from build123d import *

# Parameters (mm, degrees)
SKETCH1_W               = 10.16
SKETCH1_H               = 3.175
BOSS_EXTRUDE1_DEPTH     = 4.445
SKETCH3_OUTSIDE_W       = 14.934
SKETCH3_OUTSIDE_H       = 13.664
SKETCH3_OUTSIDE_W_2     = 10.16
SKETCH3_OUTSIDE_H_2     = 8.89
SKETCH3_OUTSIDE_W_3     = 5.08
SKETCH3_OUTSIDE_H_3     = 5.08
CUT_EXTRUDE1_DEPTH      = 1.905
CUT_EXTRUDE2_DEPTH      = 1
CUT_EXTRUDE2_DEPTH_BACK = 4.175
SKETCH6_R               = 1.5875
CUT_EXTRUDE3_DEPTH      = 0.2032


with BuildPart() as part:
    # Sketch1 → Boss-Extrude1 (new body, symmetric)
    with BuildSketch(Plane.XY):
        with Locations((0, -1.5875)):
            Rectangle(SKETCH1_W, SKETCH1_H)
    extrude(amount=BOSS_EXTRUDE1_DEPTH, both=True)

    # Sketch3 outside → Cut-Extrude1 (cut)
    with BuildSketch(Plane.XZ.offset(3.175)):
        Rectangle(SKETCH3_OUTSIDE_W, SKETCH3_OUTSIDE_H)
        Rectangle(SKETCH3_OUTSIDE_W_2, SKETCH3_OUTSIDE_H_2, mode=Mode.SUBTRACT)
        Rectangle(SKETCH3_OUTSIDE_W_3, SKETCH3_OUTSIDE_H_3)
    extrude(amount=-CUT_EXTRUDE1_DEPTH, mode=Mode.SUBTRACT)

    # Sketch5 → Cut-Extrude2 (cut, two sides)
    with BuildSketch(Plane(origin=(0, 0, 0), x_dir=(1, 0, 0), z_dir=(0, 1, 0))) as cut_extrude2_sk:
        with BuildLine():
            Line((0, 4.445), (-5.08, 4.445))
            Line((-5.08, 4.445), (-5.08, -4.445))
            Line((-5.08, -4.445), (0, -4.445))
            ThreePointArc((0, -4.445), (-4.445, 0), (0, 4.445))
        make_face()
    extrude(amount=CUT_EXTRUDE2_DEPTH, mode=Mode.SUBTRACT)
    extrude(cut_extrude2_sk.sketch, amount=-CUT_EXTRUDE2_DEPTH_BACK, mode=Mode.SUBTRACT)

    # Sketch6 → Cut-Extrude3 (cut)
    with BuildSketch(Plane.XZ.offset(1.27)):
        Circle(SKETCH6_R)
    extrude(amount=-CUT_EXTRUDE3_DEPTH, mode=Mode.SUBTRACT)


solid = part.part
Can you work these out from the model? Positions are in its coordinate system, mm. A direction names the side the tool comes from. Round coordinates to 2 decimals unless told otherwise and drop trailing zeros. Write each loop counter-clockwise with the first axis right and the second up, starting at its lowest first coordinate (ties: lowest second). Pieces come first, ordered by that corner, then holes. Notation, with made-up numbers: M 78.5,59 L 137.5,59 A21 cw 137.5,77 Z; hole C 72.25,15 d10. An arc over 180 degrees is marked long. Use a Markdown table: item, result.
Item 1: We'd pull the mould along X, two halves only. Please class faces 1 (the face through (-4.444, -1.565, 0.098)), 2 (the face through (3, -2, 4.445)), 3 (the face through (-2.54, -2, 0)): released by +X, released by -X, zero draft, split by the parting line, or undercut.
Found:
| item | result |
|---|---|
| face 1 | released by -X |
| face 2 | zero draft |
| face 3 | undercut |
Item 2: For pin 1 Ø2.5 at (x, z) = (-0.5, 0.5) entering from -Y; pin 2 Ø1.6 at (x, z) = (-0.5, 0.5) entering from -Y; pin 3 Ø0.6 at (x, y) = (-1, -2.5) entering from +Z, each with a flat end and sliding along its axis, tell me the tip position at first contact or that it passes through.
Found:
| item | result |
|---|---|
| pin 1 | stops at y = -1.27 |
| pin 2 | stops at y = -1.07 |
| pin 3 | stops at z = 4.39 |
Item 3: Which directions (+Z, -Z, +X, -X, +Y, -Y) give clear straight access to the entire face, cutting with the end or side of a thin tool? Please do faces 4 (the face through (0, -2, 2.54)), 5 (the face through (0, 0, 0)).
Found:
| item | result |
|---|---|
| face 4 | -Y |
| face 5 | +Z, -Z, +X, -X, +Y |
Item 4: If I drill on line 1 along X through (y, z) = (-2.65, -1); line 2 along X through (y, z) = (-2.8, 0.75); line 3 along Z through (x, y) = (-1.75, -2.1), over which ranges is the centre line in solid material (lowest first)? Write a range as [from, to].
Found:
| item | result |
|---|---|
| line 1 | x = [-4.33, -2.54], [2.54, 5.08] |
| line 2 | x = [-4.38, -2.54], [2.54, 5.08] |
| line 3 | z = [-4.09, -2.54], [2.54, 4.09] |
Item 5: I want a section at C-C (x = -0.5). List the corners of the cut face in (y, z) for me (3 decimals), and give its area (3 significant figures).
Found:
| item | result |
|---|---|
| outline | M -3.175,-4.417 L 0,-4.417 L 0,4.417 L -3.175,4.417 L -3.175,2.54 L -1.27,2.54 L -1.27,1.507 L -1.067,1.507 L -1.067,-1.507 L -1.27,-1.507 L -1.27,-2.54 L -3.175,-2.54 Z |
| area | 17.8 mm2 |
Item 6: I want a section at A-A (y = -1.75). List the corners of the cut face in (x, z) for me (3 decimals), and give its area (3 significant figures).
Found:
| item | result |
|---|---|
| outline | M 0,-4.445 L 5.08,-4.445 L 5.08,4.445 L 0,4.445 A4.445 ccw Z; hole M -2.54,-2.54 L 2.54,-2.54 L 2.54,2.54 L -2.54,2.54 Z |
| area | 50.4 mm2 |
Item 7: I want a section at D-D (y = -0.7). List the corners of the cut face in (x, z) for me (3 decimals).
Found:
| item | result |
|---|---|
| outline | M 0,-4.445 L 5.08,-4.445 L 5.08,4.445 L 0,4.445 A4.445 ccw Z |
